Can you work these out from the model? Positions are in its coordinate system, mm. A direction names the side the tool comes from. Coordinates: 2 decimals unless noted, no trailing zeros. Write each loop counter-clockwise with the first axis right and the second up, starting at its lowest first coordinate (ties: lowest second). Pieces come first, ordered by that corner, then holes. Notation, with made-up numbers: (-40, -23) - (16, -23) arc R18 ccw to (16, 11) - close; hole circle Ø9 at (30, -32). An arc over 180 degrees is marked (long way). Use one line per item in the form item = value. Start each with the question number.
(1) If we section it at B-B on x = -11: Please give me the cut outline in (y, z), then the cut area to 3 significant figures.
(2) If we section it at C-C on x = -16: Please give me the cut outline in (y, z), then the cut area to 3 significant figures.
(3) On a 3-axis mill with a long thin cutter (end or side, diameter ignored), from which of +Z, -Z, +X, -X, +Y, -Y can I reach the whole of each face in a straight line? I mean faces 1 (the face through (-15, 20, -5.2)), 2 (the face through (-11, 4, -5.4)), 3 (the face through (-19.6, 11, -2)). Say none if no direction works.
(4) Thinking about a two-plate mould opening in Z: for faces 4 (the face through (-15, 9, 2)), 5 (the face through (-16, -1.546, -2)), 6 (the face through (-11, 4, 0.4)), which applies, pulls with the +Z half, pulls with the -Z half, needs draft (parallel to the pull), parting line crosses it, or undercut?
(5) If we section it at D-D on y = 7.5: Please give me the cut outline in (x, z), then the cut area to 3 significant figures.
(6) If I drill on probe 1 along Z at (x, y) = (-18.9, 19.15); probe 2 along Y at (x, z) = (-18.1, -2.5); probe 3 along Y at (x, z) = (-13.75, -1.75), over which ranges is the centre line in solid material (lowest first)? Write a range as from..to.
(7) For pin 1 Ø1 at (x, z) = (-13, -6) entering from +Y; pin 2 Ø1.6 at (y, z) = (21.5, -3) entering from +X; pin 3 Ø1.5 at (y, z) = (12.5, 0) entering from +X, each with a flat end and sliding along its axis, tell me the tip position at first contact or that it passes through.
(8) If we section it at A-A on z = -2.5: Please give me the cut outline in (x, y), then the cut area to 3 significant figures.
Autodesk Inventor part; units mm, degrees
ref_plane "Work Plane1" through (0, 0, 0) normal (0, 0, 1) x (1, 0, 0)
ref_plane "Work Plane2" through (-17.5, 12.1, -5) normal (0, 0, -1) x (0, 1, 0)
ref_plane "YZ Plane" through (0, 0, 0) normal (1, 0, 0) x (0, 1, 0)
ref_plane "Work Plane1" through (0, 0, 0) normal (0, 0, 1) x (1, 0, 0)
sketch "Sketch1" plane through (0, 0, 0) normal (0, 0, 1) x (1, 0, 0)
  line L0 (-12.5, 1) -> (-12.5, -7.7)
  line L1 (-12.5, 12) -> (-12.5, 6.5)
  line L2 (-12.6, 1) -> (-12.6, -7.7)
  line L3 (-12.6, 12) -> (-12.6, 9.0456)
  arc A0 (-12.5, 1) -> (-12.5, 6.5) centre (-11.5571, 3.75) ccw
  line L4 (-12.4, 12) -> (-12.4, 6.6366)
  arc A1 (-9.4308, 1.6236) -> (-9.4308, 5.8764) centre (-11.5571, 3.75) ccw
  line L5 (-12.4, 0.8634) -> (-12.4, -7.7)
  line L6 (-9.4308, 5.8764) -> (-12.6, 9.0456)
  line L7 (-8.6562, 5.1018) -> (-1.312, 5.1018) construction
  line L8 (-9.4308, 1.6236) -> (-12.6, -1.5456)
  line L9 (-8.3764, 2.678) -> (0.7652, 2.678) construction
  line L10 (-19.6, -14) -> (-19.6, -6.5)
  line L11 (-12.6, -1.5456) -> (-19.6, -1.5456)
  line L12 (-17.5, 16.8) -> (-17.5, 21.5)
  line L13 (-12.5, 16.8) -> (-17.5, 16.8)
  line L14 (-12.6, 16.7) -> (-17.5, 16.7)
  line L15 (-12.6, 12) -> (-12.6, 16.7)
  line L16 (-17.5, 16.8) -> (-17.5, 16.7)
  line L17 (-19.6, -1.5456) -> (-19.6, 21.5)
  line L18 (-19.6, -1.5456) -> (3.4456, -1.5456) construction
  line L19 (-19.6, 21.5) -> (-17.5, 21.5)
  point P0 (0, 0)
  dimension "d0" = 0.1
  dimension "d1" = 0.1
  dimension "d2" = 0.1
  dimension "d3" = 135
  dimension "d4" = 135
  dimension "d5" = 0.1
  dimension "d6" = 90
extrude "Extrusion1" add sketch "Sketch1" along normal blind 2
sketch "Sketch2" plane through (0, 0, 0) normal (0, 0, -1) x (-1, 0, 0)
  line L0 (19.6, -1.5456) -> (12.6, -1.5456)
  line L1 (12.6, 9.0456) -> (12.6, 16.7)
  line L2 (12.6, 16.7) -> (17.5, 16.7)
  line L3 (17.5, 16.7) -> (17.5, 21.5)
  line L4 (17.5, 21.5) -> (19.6, 21.5)
  line L5 (19.6, 21.5) -> (19.6, -1.5456)
  line L6 (12.6, -1.5456) -> (12.6, 9.0456)
  point P0 (0, 0)
ref_plane "Work Plane2" through (-17.5, 12.1, -5) normal (0, 0, -1) x (0, 1, 0)
extrude "Extrusion2" add sketch "Sketch2" along normal up to surface (5 mm away)
sketch "Sketch3" plane through (-12.6, -1.5456, -5) normal (0, 0, -1) x (-1, 0, 0)
  line L0 (0, 10.5912) -> (0, 18.2456)
  line L1 (0, 18.2456) -> (4.9, 18.2456)
  line L2 (4.9, 18.2456) -> (4.9, 23.0456)
  line L3 (4.9, 23.0456) -> (7, 23.0456)
  line L4 (7, 23.0456) -> (7, 0)
  line L5 (7, 0) -> (0, 0)
  line L6 (0, 0) -> (-3.1692, 3.1692)
  arc A0 (-3.1692, 7.422) -> (-3.1692, 3.1692) centre (-1.0429, 5.2956) ccw
  line L7 (-3.1692, 7.422) -> (0, 10.5912)
  point P0 (-12.6, 1.5456)
extrude "Extrusion3" add sketch "Sketch3" along normal blind 2
sketch "Sketch4" plane through (-19.6, -1.5456, 2) normal (-1, 0, 0) x (0, 0, 1)
  line L0 (-2, 23.0456) -> (-2, 18.3456)
  line L1 (-7, 18.3456) -> (-2, 18.3456)
  line L2 (-7, 23.0456) -> (-7, 18.3456)
  line L3 (-7, 23.0456) -> (-2, 23.0456)
  line L4 (-2, 18.3456) -> (-7, 23.0456)
  circle A0 centre (-4.5, 20.6956) radius 1.5
  circle A1 centre (-4.5, 20.6956) radius 1.4
  point P0 (-2, 1.5456)
  dimension "d13" = 3
extrude "Extrusion4" cut sketch "Sketch4" against normal blind 2.75 contours A0 L4 A1 | L4 A1 A0 | A1 L4 | L4 A1
sketch "Sketch5" plane through (-19.6, -1.5456, 2) normal (-1, 0, 0) x (0, 0, 1)
  circle A0 centre (-4.5, 20.6956) radius 1.5
  line L0 (0, 23.0456) -> (0, 0)
  circle A1 centre (-4.5, 20.6956) radius 4.5
  line L1 (0, 23.0456) -> (-9, 23.0456)
  point P0 (-2, 1.5456)
  point P1 (-8.3376, 23.0456)
  point P2 (-0.6624, 23.0456)
extrude "Extrusion5" add sketch "Sketch5" against normal up to surface (2.1 mm away) contours L1 A1 picked at (-4.7918, 23.9439)
sketch "Sketch6" plane through (-19.6, -1.5456, 2) normal (-1, 0, 0) x (0, 0, 1)
  arc A0 (-0.6624, 23.0456) -> (-8.3376, 23.0456) centre (-4.5, 20.6956) ccw
  line L0 (0, 23.0456) -> (0, 0)
  line L1 (0, 23.0456) -> (-0.6624, 23.0456)
  circle A1 centre (-4.5, 20.6956) radius 4.5
  line L2 (-8.3376, 23.0456) -> (-9, 23.0456)
  line L3 (-9, 0) -> (-9, 23.0456)
  point P0 (-2, 1.5456)
  point P1 (-9, 20.6956)
  point P2 (-8.3376, 23.0456)
  point P3 (0, 20.6956)
extrude "Extrusion6" cut sketch "Sketch6" against normal blind 10 contours L1 L0 A1 | A1 L3 L2
sketch "Sketch7" plane through (-17.5, 16.7, 2) normal (1, 0, 0) x (0, 0, -1)
  line L0 (7, 4.8) -> (7, 0.1)
  line L1 (2, 4.8) -> (2, 0.1)
  line L2 (7.2, 4.8) -> (7.2, 0.1)
  line L3 (1.8, 4.8) -> (1.8, 0.1)
  arc A0 (9, 2.45) -> (0, 2.45) centre (4.5, 2.45) ccw
  line L4 (9, 2.45) -> (9, 0)
  line L5 (0, 0) -> (0, 2.45)
  line L6 (9, 0) -> (0, 0)
  line L7 (1.8, 0.1) -> (1.8, 0)
  line L8 (9, 0) -> (0, 0)
  line L9 (7.2, 0.1) -> (7.2, 0)
  line L10 (7.2, 4.8) -> (7.2, 6.05)
  line L11 (1.8, 4.8) -> (1.8, 6.05)
  point P0 (2, -16.7)
  point P1 (1.8, 0)
  dimension "d20" = 0.2
  dimension "d21" = 0.2
extrude "Extrusion7" add sketch "Sketch7" along normal up to surface (4.9 mm away) contours L10 A0 L4 L6 L9 L2 | L11 L3 L7 L6 L5 A0
sketch "Sketch8" plane through (0, 0, 0) normal (0, 0, -1) x (-1, 0, 0)
  line L0 (12.6, -1.5456) -> (12.6, 9.0456)
  line L1 (9.4308, 5.8764) -> (12.6, 9.0456)
  arc A0 (9.4308, 5.8764) -> (9.4308, 1.6236) centre (11.5571, 3.75) ccw
  line L2 (12.6, -1.5456) -> (9.4308, 1.6236)
  point P0 (0, 0)
extrude "Extrusion8" cut sketch "Sketch8" against normal blind 0.4
sketch "Sketch9" plane through (-12.6, -1.5456, -5) normal (0, 0, 1) x (1, 0, 0)
  line L0 (0, 0) -> (0, 10.5912)
  line L1 (3.1692, 3.1692) -> (0, 0)
  arc A0 (3.1692, 3.1692) -> (3.1692, 7.422) centre (1.0429, 5.2956) ccw
  line L2 (0, 10.5912) -> (3.1692, 7.422)
  point P0 (12.6, 1.5456)
extrude "Extrusion9" cut sketch "Sketch9" against normal blind 0.4
properties part number "SideCameraSlider_3DPrint"
Reported:
q1.outline = (0.05, -7) - (7.45, -7) - (7.45, -5.4) - (0.05, -5.4) - close; (0.05, 0.4) - (7.45, 0.4) - (7.45, 2) - (0.05, 2) - close
q1.area = 23.7 mm2
q2.outline = (-1.55, -7) - (19.15, -7) arc R4.5 ccw to (22.75, -5.2) - (16.7, -5.2) - (16.7, 0.2) - (22.75, 0.2) arc R4.5 ccw to (19.15, 2) - (-1.55, 2) - close
q2.area = 182 mm2
q3.face_1 = +X, +Y
q3.face_2 = +X, +Y, -Y
q3.face_3 = +Z, -Z, -X, +Y, -Y
q4.face_4 = pulls with the +Z half
q4.face_5 = needs draft
q4.face_6 = undercut
q5.outline = (-19.6, -7) - (-11.05, -7) - (-11.05, -5.4) - (-12.6, -5.4) - (-12.6, 0.4) - (-11.05, 0.4) - (-11.05, 2) - (-19.6, 2) - close
q5.area = 67.9 mm2
q6.probe_1 = -7..-4, -1..2
q6.probe_2 = -1.55..17.65, 20.65..23.65
q6.probe_3 = -1.55..16.7
q7.pin_1 = 22.5
q7.pin_2 = -17.5
q7.pin_3 = -12.6
q8.outline = (-19.6, -1.55) - (-12.6, -1.55) - (-12.6, 16.7) - (-17.5, 16.7) - (-17.5, 17.65) - (-19.6, 17.65) - close; (-19.6, 20.65) - (-17.5, 20.65) - (-17.5, 23.65) - (-19.6, 23.65) - close
q8.area = 136 mm2
